Could you check a few things on this model? Use its own coordinates, in mm. Give positions to 0.01 mm unless a question says otherwise; leave off trailing zeros. Loops run counter-clockwise (first coordinate to the right, second up) from the corner with the lowest first, then second, coordinate; pieces in that order, holes last. Notation, with made-up numbers: (-11, 45) -> (2, 45) arc R23 ccw to (2, 77) -> close; hole circle Ø8 at (85.25, 47.25). An arc over 180 degrees is marked (long way). Put each result on its own line as item: value.
```python
from build123d import *

# Parameters (mm, degrees)
F0_W     = 40
F0_H     = 40
F1_DEPTH = 4
F3_DEPTH = 25
F4_R     = 15
F5_DEPTH = 25


with BuildPart() as f1:
    # F0 (on Top) → F1 (new body)
    with BuildSketch(Plane.XY):
        with Locations((20, 20)):
            Rectangle(F0_W, F0_H)
    extrude(amount=F1_DEPTH)

    # F2 (on face) → F3 (cut)
    with BuildSketch(Plane.XY.offset(4)):
        Polygon((0, 40), (0, 31.514719), (8.485281, 40), align=None)
        Polygon((40, 40), (31.514719, 40), (40, 31.514719), align=None)
        Polygon((40, 8.485281), (31.514719, 0), (40, 0), align=None)
        Polygon((8.485281, 0), (0, 8.485281), (0, 0), align=None)
    extrude(amount=-F3_DEPTH, mode=Mode.SUBTRACT)

    # F4 (on face) → F5 (cut)
    with BuildSketch(Plane.XY.offset(4)):
        with Locations((20, 20)):
            Circle(F4_R)
    extrude(amount=-F5_DEPTH, mode=Mode.SUBTRACT)


solid = f1.part
```
1. I'm going to push flat-ended pins straight in: pin 1 (6 mm diameter, centred on x = 9.5, y = 21, fed in from -Z); pin 2 (1.5 mm diameter, centred on y = 35, z = 3, fed in from +X). Where does each tip first touch, or does it pass through?
Recorded:
pin 1: passes through
pin 2: stops at x = 37.26
2. I need wall thicknesses on line 1 (Y direction, x = 20, z = 2.2); line 2 (X direction, y = 14, z = 3.1); line 3 (Y direction, x = 12.5, z = 3.2). Which ranges of each line are inside material? Lowest first, please.
Recorded:
line 1: y = 0 to 5, 35 to 40
line 2: x = 0 to 6.25, 33.75 to 40
line 3: y = 0 to 7.01, 32.99 to 40
3. If we section it at B-B (y = 20): List the corners of the cut face in (x, z) for me, then the cut area to 3 significant figures.
Recorded:
outline: (0, 0) -> (5, 0) -> (5, 4) -> (0, 4) -> close; (35, 0) -> (40, 0) -> (40, 4) -> (35, 4) -> close
area: 40.0 mm^2
4. Thinking about a two-plate mould opening in Y: for faces 1 (the face through (20, 0, 2)), 2 (the face through (16.748, 5.357, 2.028)), 3 (the face through (29, 7, 0)), which applies, pulls with the +Y half, pulls with the -Y half, needs draft (parallel to the pull), parting line crosses it, or undercut?
Recorded:
face 1: pulls with the -Y half
face 2: undercut
face 3: needs draft
5. If we section it at C-C (x = 26.5): List the corners of the cut face in (y, z) for me, then the cut area to 3 significant figures.
Recorded:
outline: (0, 0) -> (6.48, 0) -> (6.48, 4) -> (0, 4) -> close; (33.52, 0) -> (40, 0) -> (40, 4) -> (33.52, 4) -> close
area: 51.9 mm^2
6. If we section it at A-A (z = 3.45): List the corners of the cut face in (x, y) for me.
Recorded:
outline: (0, 8.49) -> (8.49, 0) -> (31.51, 0) -> (40, 8.49) -> (40, 31.51) -> (31.51, 40) -> (8.49, 40) -> (0, 31.51) -> close; hole circle Ø30 at (20, 20)
